Read the model definition and answer for the solid it produces. Units are mm, in the model's axes. Face numbers are marked on the shaded views. A direction names the side the tool comes from. Give positions to 0.01 mm unless a question says otherwise; leave off trailing zeros. Order: outer loops, then holes, each group sorted by start corner. A loop starts at its lowest first (then second) coordinate and runs counter-clockwise, first axis right, second up. Notation, with made-up numbers: M -35.75,42.5 L -22.75,42.5 A29 cw -22.75,75.5 Z; hole C -19.5,81.5 d8. An arc over 180 degrees is marked long. Write item = value, one per line. Start each with the question number.
from build123d import *

# Parameters (mm, degrees)
SKETCH067_R     = 2.25
PAD050_DEPTH    = 3.5
PAD051_DEPTH    = 51
PAD052_DEPTH    = 3
CHAMFER005_SIZE = 2
SKETCH070_R     = 4
SKETCH070_W     = 66
SKETCH070_H     = 42.5
SKETCH070_W_2   = 10
SKETCH070_H_2   = 25
POCKET033_DEPTH = 80.001
SKETCH071_W     = 3.5
SKETCH071_H     = 10
PAD053_DEPTH    = 8


with BuildPart() as part:
    # Sketch067 → Pad050 (new body)
    with BuildSketch(Plane.XZ):
        with BuildLine():
            Line((55.25, 24), (-55.25, 24))
            Line((-55.25, 24), (-55.25, 14))
            Line((-55.25, 14), (-10, 14))
            Line((-10, 14), (-10, -42.5))
            Line((-10, -42.5), (-55.25, -42.5))
            Line((-55.25, -42.5), (-55.25, -45))
            ThreePointArc((-55.25, -45), (-52.028175, -52.778175), (-44.25, -56))
            Line((44.25, -56), (-44.25, -56))
            ThreePointArc((44.25, -56), (52.028175, -52.778175), (55.25, -45))
            Line((55.25, -42.5), (55.25, -45))
            Line((10, -42.5), (55.25, -42.5))
            Line((10, 14), (10, -42.5))
            Line((55.25, 14), (10, 14))
            Line((55.25, 24), (55.25, 14))
        make_face()
        Circle(SKETCH067_R, mode=Mode.SUBTRACT)
        with Locations((0, -30)):
            Circle(SKETCH067_R, mode=Mode.SUBTRACT)
    extrude(amount=PAD050_DEPTH)

    # Sketch068 (on Face17 of Pad050) → Pad051 (join)
    with BuildSketch(Plane(origin=(0, 0, 0), x_dir=(1, 0, 0), z_dir=(0, 1, 0))):
        with BuildLine():
            Line((-55.25, 45), (-55.25, 42.5))
            Line((-55.25, 42.5), (-51.75, 42.5))
            Line((-51.75, 42.5), (-51.75, 45))
            ThreePointArc((-44.25, 52.5), (-49.553301, 50.303301), (-51.75, 45))
            Line((-44.25, 52.5), (44.25, 52.5))
            ThreePointArc((51.75, 45), (49.553301, 50.303301), (44.25, 52.5))
            Line((51.75, 42.5), (51.75, 45))
            Line((55.25, 42.5), (51.75, 42.5))
            Line((55.25, 45), (55.25, 42.5))
            ThreePointArc((55.25, 45), (52.028175, 52.778175), (44.25, 56))
            Line((-44.25, 56), (44.25, 56))
            ThreePointArc((-44.25, 56), (-52.028175, 52.778175), (-55.25, 45))
        make_face()
    extrude(amount=PAD051_DEPTH)

    # Sketch069 (on Face17 of Pad051) → Pad052 (join)
    with BuildSketch(Plane(origin=(0, 51, 0), x_dir=(1, 0, 0), z_dir=(0, 1, 0))):
        with BuildLine():
            Line((-55.25, 45), (-55.25, 42.5))
            Line((-55.25, 42.5), (-49.75, 42.5))
            ThreePointArc((-49.75, 42.5), (-47.982233, 43.232233), (-47.25, 45))
            ThreePointArc((-44.25, 48), (-46.37132, 47.12132), (-47.25, 45))
            Line((-44.25, 48), (44.25, 48))
            ThreePointArc((47.25, 45), (46.37132, 47.12132), (44.25, 48))
            ThreePointArc((47.25, 45), (47.982233, 43.232233), (49.75, 42.5))
            Line((55.25, 42.5), (49.75, 42.5))
            Line((55.25, 45), (55.25, 42.5))
            ThreePointArc((55.25, 45), (52.028175, 52.778175), (44.25, 56))
            Line((-44.25, 56), (44.25, 56))
            ThreePointArc((-44.25, 56), (-52.028175, 52.778175), (-55.25, 45))
        make_face()
    extrude(amount=PAD052_DEPTH)

    # Chamfer005
    chamfer005_edges = [part.edges().sort_by_distance(p)[0] for p in [
        (-2.25, 0, -30),
        (-2.25, 0, 0),
    ]]
    chamfer(chamfer005_edges, length=CHAMFER005_SIZE)

    # Sketch070 (on Face28 of Chamfer005) → Pocket033 (cut, through all)
    with BuildSketch(Plane(origin=(0, 0, -56), x_dir=(1, 0, 0), z_dir=(0, 0, -1))):
        with Locations((-41, -30.5)):
            Circle(SKETCH070_R)
        with Locations((0, -25.25)):
            Rectangle(SKETCH070_W, SKETCH070_H)
        with Locations((39.5, -25)):
            Rectangle(SKETCH070_W_2, SKETCH070_H_2)
    extrude(amount=-POCKET033_DEPTH, mode=Mode.SUBTRACT)

    # Sketch071 (on Face4 of Pad051) → Pad053 (join)
    with BuildSketch(Plane(origin=(0, 0, 0), x_dir=(1, 0, 0), z_dir=(0, 1, 0))):
        with Locations((-53.5, -19)):
            Rectangle(SKETCH071_W, SKETCH071_H)
        with Locations((53.5, -19)):
            Rectangle(SKETCH071_W, SKETCH071_H)
    extrude(amount=PAD053_DEPTH)


solid = part.part
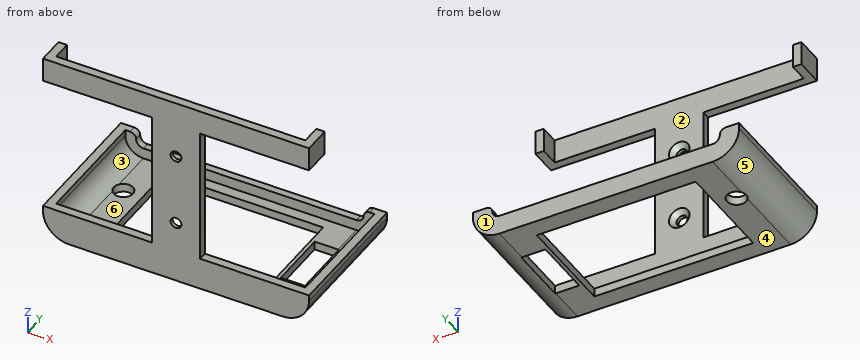
1) Find section C-C on z = 0. Determine the outline of the cut face in (x, y), plus the area to 4 significant figures.
2) Find section A-A on y = 41.5. Determine the outline of the cut face in (x, z), plus the area to 3 significant figures.
3) Each of these flat-tipped pins is pushed along its axis until it touches: P1, Ø1, axis at y = -1.5, z = -7.5, coming from the +X side; P2, Ø4, axis at x = 0, z = 0, coming from the +Y side; P3, Ø1.8, axis at y = 21.5, z = -54, coming from the +X side; P4, Ø4, axis at y = 27.5, z = -55, coming from the +X side. Where does it stop, or does it pass through?
4) Find section D-D on x = -39.5. Determine the outline of the cut face in (y, z).
5) Find the intervals of material crossed by probe 1 along Z at (x, y) = (0, -2.6); probe 2 along Y at (x, z) = (18, -51.5); probe 3 along X at (y, z) = (30, -54), in increasing order. Write a range as [from, to].
6) Find section B-B on x = 0. Determine the outline of the cut face in (y, z).
7) For the marked faces 1 and 2, determine the directions among +Z, -Z, +X, -X, +Y, -Y from which every point of the face is accessible in a straight line to the end or side of a thin tool.
8) For a pull along X with two mould halves and no side action, classify the marked faces 3, 4, 5 and 6 as pulls with the +X half, pulls with the -X half, needs draft (parallel to the pull), parting line crosses it, or undercut.
Numbers:
q1.outline = M -10,-3.5 L -2.25,-3.5 L -2.25,-2 L -4.25,0 L -10,0 Z; M 2.25,-3.5 L 10,-3.5 L 10,0 L 4.25,0 L 2.25,-2 Z
q1.area = 50.25 mm2
q2.outline = M -55.25,-45 A11 ccw -44.25,-56 L -33,-56 L -33,-52.5 L -44.25,-52.5 A7.5 cw -51.75,-45 L -51.75,-42.5 L -55.25,-42.5 Z; M 33,-56 L 44.25,-56 A11 ccw 55.25,-45 L 55.25,-42.5 L 51.75,-42.5 L 51.75,-45 A7.5 cw 44.25,-52.5 L 33,-52.5 Z
q2.area = 198 mm2
q3.P1 = 10
q3.P2 = through
q3.P3 = 51.69
q3.P4 = 51.8
q4.outline = M -3.5,-56 L 26.79,-56 L 26.79,-52.5 L 0,-52.5 L 0,-42.5 L -3.5,-42.5 Z; M -3.5,14 L 0,14 L 0,24 L -3.5,24 Z; M 34.21,-56 L 54,-56 L 54,-48 L 51,-48 L 51,-52.5 L 34.21,-52.5 Z
q5.probe_1 = [-56, -32.25], [-27.75, -2.25], [2.25, 24]
q5.probe_2 = [-3.5, 0], [51, 54]
q5.probe_3 = [-50.57, -44.97], [-37.03, -33], [33, 34.5], [44.5, 50.57]
q6.outline = M -3.5,-56 L 4,-56 L 4,-52.5 L 0,-52.5 L 0,-34.25 L -2,-32.25 L -3.5,-32.25 Z; M -3.5,-27.75 L -2,-27.75 L 0,-25.75 L 0,-4.25 L -2,-2.25 L -3.5,-2.25 Z; M -3.5,2.25 L -2,2.25 L 0,4.25 L 0,24 L -3.5,24 Z; M 46.5,-56 L 54,-56 L 54,-48 L 51,-48 L 51,-52.5 L 46.5,-52.5 Z
q7.face_1 = +Z, -Z, +X, -X, +Y
q7.face_2 = +Z
q8.face_3 = undercut
q8.face_4 = needs draft
q8.face_5 = pulls with the -X half
q8.face_6 = undercut
